from build123d import *

# Parameters (mm, degrees)
F0_W     = 50.8
F0_H     = 25.4
F0_W_2   = 47.625
F0_H_2   = 22.225
F1_DEPTH = 508
F3_D     = 5.1054
F5_D     = 5.1054


with BuildPart() as f1:
    # F0 (on Top) → F1 (new body)
    with BuildSketch(Plane.XY):
        Rectangle(F0_W, F0_H)
        Rectangle(F0_W_2, F0_H_2, mode=Mode.SUBTRACT)
    extrude(amount=F1_DEPTH)

    # F3 (through all)
    with Locations(Plane.XZ.offset(12.7)):
        with Locations((-12.7, 317.5), (-12.7, 342.9), (12.7, 342.9), (12.7, 317.5), (12.7, 292.1), (12.7, 266.7), (-12.7, 266.7), (-12.7, 292.1), (12.7, 114.3), (-12.7, 114.3), (-12.7, 139.7), (12.7, 139.7), (12.7, 165.1), (-12.7, 165.1), (-12.7, 190.5), (12.7, 190.5), (-12.7, 215.9), (12.7, 241.3), (-12.7, 241.3), (12.7, 215.9), (-12.7, 419.1), (-12.7, 469.9), (12.7, 469.9), (12.7, 419.1), (12.7, 444.5), (-12.7, 444.5), (-12.7, 393.7), (12.7, 393.7), (12.7, 368.3), (-12.7, 368.3), (12.7, 63.5), (12.7, 88.9), (12.7, 12.7), (12.7, 38.1), (-12.7, 12.7), (-12.7, 38.1), (-12.7, 63.5), (-12.7, 88.9), (-12.7, 495.3), (12.7, 495.3)):
            Hole(F3_D / 2)

    # F5 (through all)
    with Locations(Plane.YZ.offset(25.4)):
        with Locations((0, 38.1), (0, 12.7), (0, 88.9), (0, 63.5), (0, 215.9), (0, 190.5), (0, 165.1), (0, 139.7), (0, 114.3), (0, 444.5), (0, 469.9), (0, 419.1), (0, 317.5), (0, 342.9), (0, 368.3), (0, 393.7), (0, 266.7), (0, 292.1), (0, 241.3), (0, 495.3)):
            Hole(F5_D / 2)


solid = f1.part
Part model, mm, in its own coordinate system. A direction names the side the tool comes from. Coordinates: 2 decimals unless noted, no trailing zeros. Order: outer loops, then holes, each group sorted by start corner. A loop starts at its lowest first (then second) coordinate and runs counter-clockwise, first axis right, second up.
(1) Pin check, flat tip, straight feed: pin 1 Ø4.5 at (y, z) = (0, 444.5) entering from -X. Stop position of the tip, or through.
Check sheet entries:
pin 1: passes through
(2) Probe L1, parallel to X at y = 11.6, z = 342.9; L2, parallel to X at y = 2, z = 54; L3, parallel to Y at x = -12.5, z = 403.5. List the from-to ranges inside material, lowest first.
Check sheet entries:
L1: x = -25.4 to -15.25, -10.15 to 10.15, 15.25 to 25.4
L2: x = -25.4 to -23.81, 23.81 to 25.4
L3: y = -12.7 to -11.11, 11.11 to 12.7
(3) Slice it at A-A, the plane y = -7. Write the cut outline in (x, z), and give its area (3 significant figures).
Check sheet entries:
outline: (-25.4, 0) - (-23.81, 0) - (-23.81, 508) - (-25.4, 508) - close; (23.81, 0) - (25.4, 0) - (25.4, 508) - (23.81, 508) - close
area: 1,610 mm2
(4) Slice it at B-B, the plane z = 205. Write the cut outline in (x, y).
Check sheet entries:
outline: (-25.4, -12.7) - (25.4, -12.7) - (25.4, 12.7) - (-25.4, 12.7) - close; hole (-23.81, -11.11) - (23.81, -11.11) - (23.81, 11.11) - (-23.81, 11.11) - close
(5) Slice it at C-C, the plane x = -5.5. Write the cut outline in (y, z), and give its area (3 significant figures).
Check sheet entries:
outline: (-12.7, 0) - (-11.11, 0) - (-11.11, 508) - (-12.7, 508) - close; (11.11, 0) - (12.7, 0) - (12.7, 508) - (11.11, 508) - close
area: 1,610 mm2
(6) Pull direction X, two halves, no side cores. Call faces 3 (the face through (-23.812, 0, 250)), 4 (the face through (0, 12.7, 250)), 5 (the face through (25.4, 0, 250)): pulls with the +X half, pulls with the -X half, needs draft (parallel to the pull), parting line crosses it, or undercut.
Check sheet entries:
face 3: undercut
face 4: needs draft
face 5: pulls with the +X half
(7) Tool access for faces 1 (the face through (0, -12.7, 250)), 2 (the face through (0, 11.112, 250)): list every direction of +Z, -Z, +X, -X, +Y, -Y with a clear straight run to the whole face (end or side of a thin tool).
Check sheet entries:
face 1: +Z, -Z, +X, -X, -Y
face 2: +Z, -Z
